Read the model definition and answer for the solid it produces. Units are mm, in the model's axes. A direction names the side the tool comes from. Give positions to 0.01 mm unless a question says otherwise; leave off trailing zeros. Write each loop counter-clockwise with the first axis right and the second up, starting at its lowest first coordinate (ties: lowest second). Pieces come first, ordered by that corner, then holes. Notation, with made-up numbers: (3, 30) -> (59, 30) arc R20 cw to (59, 65) -> close; hole circle Ø8 at (13, -13.75). An arc over 180 degrees is marked (long way). Put each result on its own line as item: value. Start each with the question number.
from build123d import *

# Parameters (mm, degrees)
SKETCH1_R                                         = 11.43
BOSS_EXTRUDE1_DEPTH                               = 4.7625
F_10_32_TAPPED_HOLE1_D                            = 4.0386
F_10_CLEARANCE_HOLE1_D                            = 4.9784
FILLET1_R                                         = 5.08
CSK_FOR_6_FLAT_HEAD_MACHINE_SCREW_100_D           = 3.7973
CSK_FOR_6_FLAT_HEAD_MACHINE_SCREW_100_CSINK_D     = 7.0866
CSK_FOR_6_FLAT_HEAD_MACHINE_SCREW_100_CSINK_ANGLE = 100


with BuildPart() as part:
    # Sketch1 → Boss-Extrude1 (new body)
    with BuildSketch(Plane(origin=(0, 0, 0), x_dir=(0, 0, -1), z_dir=(1, 0, 0))):
        with BuildLine():
            Line((-25.4, 25.4), (-25.4, -3.844624666))
            ThreePointArc((-25.4, -3.844624666), (-26.750820168, -7.294206927), (-30.084888889, -8.909235926))
            ThreePointArc((-30.084888889, -8.909235926), (-35.941, -15.24), (-30.084888889, -21.570764074))
            ThreePointArc((-30.084888889, -21.570764074), (-27.201538941, -22.75489945), (-25.552500859, -25.4))
            Line((-25.552500859, -25.4), (-25.4, -25.4))
            Line((-25.4, -25.4), (25.4, -25.4))
            Line((25.4, -25.4), (30.1625, -25.4))
            ThreePointArc((30.1625, -25.4), (36.511887391, -19.138202954), (30.338888889, -12.702450318))
            ThreePointArc((30.338888889, -12.702450318), (26.83834897, -11.166271352), (25.4, -7.624410573))
            Line((25.4, -7.624410573), (25.4, 7.624410573))
            ThreePointArc((25.4, 7.624410573), (26.83834897, 11.166271352), (30.338888889, 12.702450318))
            ThreePointArc((30.338888889, 12.702450318), (36.511887391, 19.138202954), (30.1625, 25.4))
            Line((30.1625, 25.4), (25.4, 25.4))
            Line((25.4, 25.4), (-25.4, 25.4))
        make_face()
        with Locations(Location((0, 0, 0), (0, 0, 180))):
            Circle(SKETCH1_R, mode=Mode.SUBTRACT)
    extrude(amount=BOSS_EXTRUDE1_DEPTH)

    # #10-32 Tapped Hole1 (through all)
    with Locations(Plane(origin=(4.7625, 0, 0), x_dir=(0, 0, -1), z_dir=(1, 0, 0))):
        with Locations((-10.9601, 10.9601), (-10.9601, -10.9601), (10.9601, -10.9601), (10.9601, 10.9601)):
            Hole(F_10_32_TAPPED_HOLE1_D / 2)

    # #10 Clearance Hole1 (through all)
    with Locations(Plane(origin=(4.7625, 0, 0), x_dir=(0, 0, -1), z_dir=(1, 0, 0))):
        with Locations((-29.591, -15.24), (30.1625, 19.05), (30.1625, -19.05)):
            Hole(F_10_CLEARANCE_HOLE1_D / 2)

    # Fillet1
    fillet1_edges = [part.edges().sort_by_distance(p)[0] for p in [
        (2.38125, -25.4, 25.552500859),
        (2.38125, 25.4, 25.4),
    ]]
    fillet(fillet1_edges, radius=FILLET1_R)

    # CSK for #6 Flat Head Machine Screw (100)1 (through all)
    with Locations(Plane(origin=(0, 10.9601, 10.9601), x_dir=(0, 0, -1), z_dir=(-1, 0, 0))):
        with Locations((0, 0), (0, 21.9202), (21.9202, 21.9202), (21.9202, 0)):
            CounterSinkHole(CSK_FOR_6_FLAT_HEAD_MACHINE_SCREW_100_D / 2, CSK_FOR_6_FLAT_HEAD_MACHINE_SCREW_100_CSINK_D / 2, counter_sink_angle=CSK_FOR_6_FLAT_HEAD_MACHINE_SCREW_100_CSINK_ANGLE)


solid = part.part
1) For a pull along Y with two mould halves and no side action, classify faces 4 (the face through (2.415, 23.872, 23.951)), 5 (the face through (2.348, -16.755, 27.616)), 6 (the face through (4.762, 12, 0)) as pulls with the +Y half, pulls with the -Y half, needs draft (parallel to the pull), parting line crosses it, or undercut.
2) A cutting plane is placed at D-D on z = 23.5. Give the vertices of the cut face in (x, y), and give its area (3 significant figures).
3) A cutting plane is placed at C-C on x = 3.4. State how many separate pieces and enclosed holes the cut face has, and give its area (3 significant figures).
4) Each of these flat-tipped pins is pushed along its axis until it touches: pin 1 Ø3 at (y, z) = (-10.96, -10.96) entering from -X; pin 2 Ø1.5 at (x, y) = (2.5, -7) entering from +Z; pin 3 Ø1.4 at (x, y) = (2.5, 9.5) entering from +Z. Where does it stop, or does it pass through?
5) A cutting plane is placed at A-A on y = 0. Give the vertices of the cut face in (x, z), and give its area (3 significant figures).
6) Straight lines are drawn through the part: line 1 (Y direction, x = 0.4, z = -11.5); line 2 (Y direction, x = 1.05, z = -9.5); line 3 (Y direction, x = 1.25, z = -9.5). For each, find the intervals that lie inside material, in ascending order. Write a range as [from, to].
7) For faces 1 (the face through (2.35, -11.21, -26.88)), 2 (the face through (2, 8, 25.4)), 3 (the face through (2.348, 6.955, -9.07)), determine the directions among +Z, -Z, +X, -X, +Y, -Y from which every point of the face is accessible in a straight line to the end or side of a thin tool.
Results found:
1. face 4: pulls with the +Y half
1. face 5: undercut
1. face 6: needs draft
2. outline: (0, -25.3) -> (4.76, -25.3) -> (4.76, 24.28) -> (0, 24.28) -> close
2. area: 236 mm²
3. separate pieces: 1
3. enclosed holes: 8
3. area: 2,440 mm²
4. pin 1: passes through
4. pin 2: stops at z = 27.23
4. pin 3: stops at z = 25.4
5. outline: (0, -25.4) -> (4.76, -25.4) -> (4.76, -11.43) -> (0, -11.43) -> close; (0, 11.43) -> (4.76, 11.43) -> (4.76, 25.4) -> (0, 25.4) -> close
5. area: 133 mm²
6. line 1: y = [-25.4, -13.98], [-7.94, 7.94], [13.98, 25.4]
6. line 2: y = [-25.4, -12.73], [-9.19, -6.36], [6.36, 9.19], [12.73, 25.4]
6. line 3: y = [-25.4, -12.4], [-9.52, -6.36], [6.36, 9.52], [12.4, 25.4]
7. face 1: -Z, +X, -X
7. face 2: +Z, +X, -X, +Y
7. face 3: +X, -X
